Input: part model. Units: mm. Frame: model coordinates. Face numbers are marked on the shaded views. A direction names the side the tool comes from. Coordinates: 2 decimals unless noted, no trailing zeros. Order: outer loops, then holes, each group sorted by start corner. A loop starts at its lowest first (then second) coordinate and runs counter-clockwise, first axis right, second up. Notation, with made-up numbers: (14, 57) -> (62, 57) arc R28 ccw to (62, 76) -> close; hole circle Ø7 at (-1.5, 52). An arc over 180 degrees is marked (long way). Answer as CSV lines item,"result".
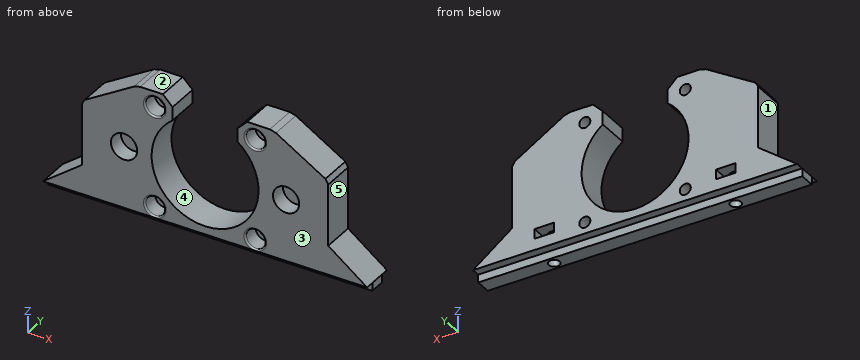
from build123d import *

# Parameters (mm, degrees)
SKETCH012_R             = 1.7
PAD001_DEPTH            = 10
SKETCH021_W             = 2.45
SKETCH021_H             = 4.8
PAD002_DEPTH            = 100
SKETCH020_R             = 4.05
SKETCH020_R_2           = 3
POCKET014_DEPTH         = 5
SKETCH013_R             = 1.7
POCKET016_DEPTH         = 22
POCKET015_DEPTH         = 3
FILLET_R                = 0.5
CHAMFER_SIZE            = 1
BODY001_ROLL_ANGLE      = 90
BODY001_PLACEMENT_ANGLE = 180


with BuildPart() as part:
    # Sketch012 → Pad001 (new body)
    with BuildSketch(Plane.XY):
        with BuildLine():
            Line((29, 48.75), (12, 38.5))
            Line((12, 38.5), (12, 18.5))
            Line((12, 18.5), (0, 9.49))
            Line((0, 9.49), (100, 9.49))
            Line((88, 18.5), (100, 9.49))
            Line((88, 18.5), (88, 38.5))
            Line((88, 38.5), (71, 48.75))
            Line((63, 48.75), (71, 48.75))
            Line((63, 48.75), (60, 45.75))
            Line((60, 45.75), (60, 41.624405))
            ThreePointArc((40, 41.624405), (50, 12), (60, 41.624405))
            Line((40, 45.75), (40, 41.624405))
            Line((37, 48.75), (40, 45.75))
            Line((29, 48.75), (37, 48.75))
        make_face()
        with Locations((34.5, 44)):
            Circle(SKETCH012_R, mode=Mode.SUBTRACT)
        with Locations((34.5, 13)):
            Circle(SKETCH012_R, mode=Mode.SUBTRACT)
        with Locations((65.5, 44)):
            Circle(SKETCH012_R, mode=Mode.SUBTRACT)
        with Locations((65.5, 13)):
            Circle(SKETCH012_R, mode=Mode.SUBTRACT)
    extrude(amount=PAD001_DEPTH)

    # Sketch021 → Pad002 (join)
    with BuildSketch(Plane.YZ):
        with Locations((8.275, 5)):
            Rectangle(SKETCH021_W, SKETCH021_H)
    extrude(amount=PAD002_DEPTH)

    # Sketch020 → Pocket014 (cut)
    with BuildSketch(Plane.XY):
        with Locations((25, 28.5)):
            Circle(SKETCH020_R)
        with Locations((75, 28.5)):
            Circle(SKETCH020_R)
        with Locations((34.5, 44)):
            Circle(SKETCH020_R_2)
        with Locations((65.5, 44)):
            Circle(SKETCH020_R_2)
        with Locations((65.5, 13)):
            Circle(SKETCH020_R_2)
        with Locations((34.5, 13)):
            Circle(SKETCH020_R_2)
    extrude(amount=POCKET014_DEPTH, mode=Mode.SUBTRACT)

    # Sketch013 → Pocket016 (cut)
    with BuildSketch(Plane.XZ):
        with Locations((22, 5)):
            Circle(SKETCH013_R)
        with Locations((78, 5)):
            Circle(SKETCH013_R)
    extrude(amount=-POCKET016_DEPTH, mode=Mode.SUBTRACT)

    # Sketch014 → Pocket015 (cut)
    with BuildSketch(Plane.XZ.offset(-13)):
        Polygon((25.031089, 3.25), (25.031089, 6.75), (25.031089, 10.75), (18.968911, 10.75), (18.968911, 6.75), (18.968911, 3.25), (22, 1.5), align=None)
        Polygon((81.031089, 3.25), (81.031089, 6.75), (81.031089, 10.75), (74.968911, 10.75), (74.968911, 6.75), (74.968911, 3.25), (78, 1.5), align=None)
    extrude(amount=-POCKET015_DEPTH, mode=Mode.SUBTRACT)

    # Fillet
    fillet_edges = [part.edges().sort_by_distance(p)[0] for p in [
        (62.5, 13, 0),
        (62.5, 44, 0),
        (31.5, 44, 0),
        (31.5, 13, 0),
    ]]
    fillet(fillet_edges, radius=FILLET_R)

    # Chamfer
    chamfer_edges = [part.edges().sort_by_distance(p)[0] for p in [
        (88, 38.5, 5),
        (71, 48.75, 5),
        (29, 48.75, 5),
        (12, 38.5, 5),
    ]]
    chamfer(chamfer_edges, length=CHAMFER_SIZE)


with BuildPart() as part_1:
    # Body001 roll: moved
    add(part.part.rotate(Axis((0, 0, 0), (1, 0, 0)), BODY001_ROLL_ANGLE))


with BuildPart() as part_2:
    # Body001 placement: moved
    add(part_1.part.moved(Location((240, 54, 0))).rotate(Axis((240, 54, 0), (0, 0, 1)), BODY001_PLACEMENT_ANGLE))


solid = part_2.part
1. Contact query for flat-ended pins moving along their axis: pin 1 (1.5 mm diameter, centred on x = 154.5, y = 60, fed in from +Z); pin 2 (4 mm diameter, centred on y = 55, z = 31.5, fed in from +X); pin 3 (3 mm diameter, centred on x = 218, y = 59, fed in from -Z). Output: stop coordinate, or through.
Findings:
pin 1,"stops at z = 40.46"
pin 2,"stops at x = 228"
pin 3,"stops at z = 22"
2. Mould query, pull axis X, two halves, no side actions, for the marked faces 3, 4 and 5. Classes: released by +X, released by -X, zero draft, split by the parting line, or undercut.
Findings:
face 3,"zero draft"
face 4,"undercut"
face 5,"released by +X"
3. Ray query, line 1 along X through (y, z) = (63.5, 44); line 2 along X through (y, z) = (55.25, 26); line 3 along Y through (x, z) = (218, 17.9). Return the intervals inside material, ascending.
Findings:
line 1,"x = 161.12 to 172.8, 176.2 to 180, 200 to 203.8, 207.2 to 218.88"
line 2,"x = 152 to 161.81, 168.19 to 173.69, 206.31 to 211.81, 218.19 to 228"
line 3,"y = 54 to 57.3, 60.7 to 64"
4. Cut plane D-D (z = 31.5). Return the cut outline in (x, y), plus the area to 3 significant figures.
Findings:
outline,"(152, 54) -> (162.28, 54) -> (162.28, 59) -> (167.72, 59) -> (167.72, 54) -> (173.78, 54) -> (173.78, 64) -> (152, 64) -> close; (206.22, 54) -> (212.28, 54) -> (212.28, 59) -> (217.72, 59) -> (217.72, 54) -> (228, 54) -> (228, 64) -> (206.22, 64) -> close"
area,"381 mm2"
5. Reachability of the marked faces 1 and 2 from +Z, -Z, +X, -X, +Y, -Y: full face, straight path, thin tool, end or side. Return the list, or none.
Findings:
face 1,"+Z, -X, +Y, -Y"
face 2,"+Z, +X, -X, +Y, -Y"
6. Cut plane A-A (y = 62.75). State how many separate pieces and enclosed holes the cut face has, plus the area to 3 significant figures.
Findings:
separate pieces,"1"
enclosed holes,"6"
area,"1,880 mm2"
7. Cut plane B-B (z = 44). Return the cut outline in (x, y), plus the area to 3 significant figures.
Findings:
outline,"(161.12, 54) -> (171, 54) arc R0.5 ccw to (171.5, 54.5) -> (171.5, 59) -> (172.8, 59) -> (172.8, 64) -> (161.12, 64) -> close; (176.2, 59) -> (177.5, 59) -> (177.5, 54.5) arc R0.5 ccw to (178, 54) -> (180, 54) -> (180, 64) -> (176.2, 64) -> close; (200, 54) -> (202, 54) arc R0.5 ccw to (202.5, 54.5) -> (202.5, 59) -> (203.8, 59) -> (203.8, 64) -> (200, 64) -> close; (207.2, 59) -> (208.5, 59) -> (208.5, 54.5) arc R0.5 ccw to (209, 54) -> (218.88, 54) -> (218.88, 64) -> (207.2, 64) -> close"
area,"283 mm2"
